Print and shaded views of the part. All mm, measured from the part's lowest x, y and z. Coordinates: 2 decimals unless noted, no trailing zeros. Order: outer loops, then holes, each group sorted by start corner. A loop starts at its lowest first (then second) coordinate and runs counter-clockwise, first axis right, second up.
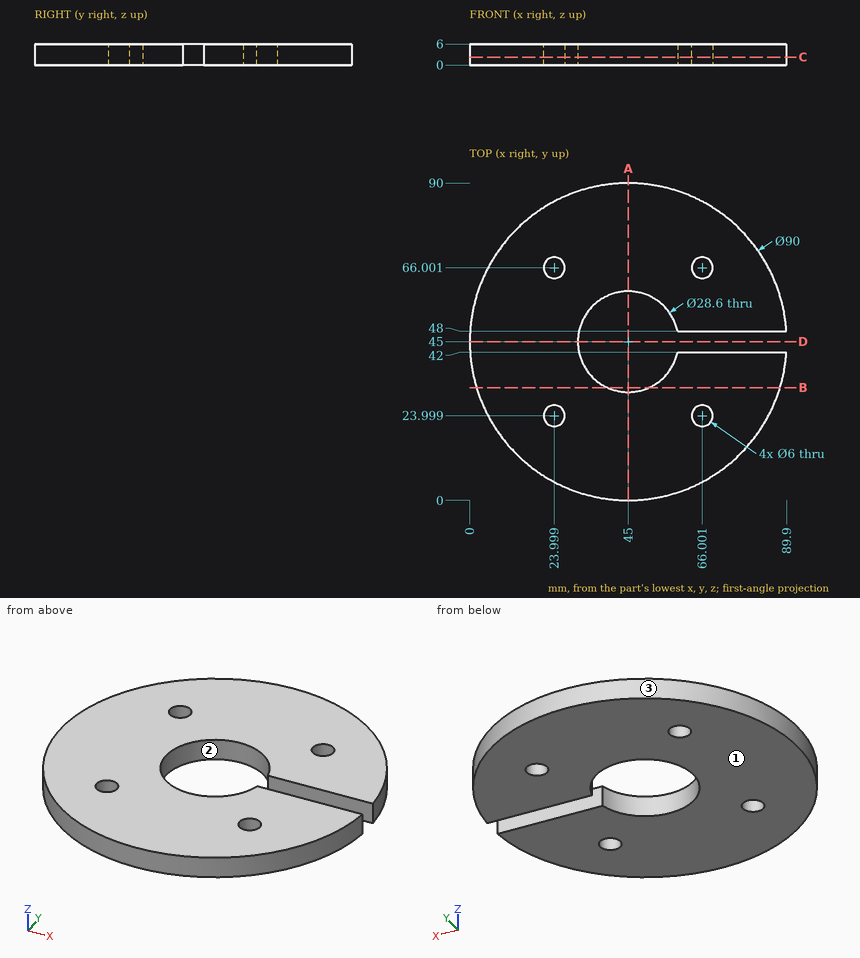
Q1. Mould opens along Y. For the marked faces 1, 2 and 3 say: pulls with the +Y half, pulls with the -Y half, needs draft (parallel to the pull), parting line crosses it, or undercut.
Established:
face 1: needs draft
face 2: undercut
face 3: parting line crosses it
Q2. Cut at A-A, the plane x = 45. List the corners of the cut face in (y, z), plus the area to 3 significant figures.
Established:
outline: (0, 0) - (30.7, 0) - (30.7, 6) - (0, 6) - close; (59.3, 0) - (90, 0) - (90, 6) - (59.3, 6) - close
area: 368 mm2
Q3. Cut at C-C, the plane z = 2.3. List the corners of the cut face in (x, y).
Established:
outline: (58.98, 42) arc R14.3 cw (long way) to (58.98, 48) - (89.9, 48) arc R45 ccw (long way) to (89.9, 42) - close; hole circle Ø6 at (24, 24); hole circle Ø6 at (24, 66); hole circle Ø6 at (66, 24); hole circle Ø6 at (66, 66)
Q4. Cut at D-D, the plane y = 45. List the corners of the cut face in (x, z), plus the area to 3 significant figures.
Established:
outline: (0, 0) - (30.7, 0) - (30.7, 6) - (0, 6) - close
area: 184 mm2
Q5. Cut at B-B, the plane y = 32. List the corners of the cut face in (x, z).
Established:
outline: (1.92, 0) - (39.04, 0) - (39.04, 6) - (1.92, 6) - close; (50.96, 0) - (88.08, 0) - (88.08, 6) - (50.96, 6) - close
Q6. Probe line 1 (X direction, y = 65, z = 0.6); line 2 (X direction, y = 45, z = 3.55); line 3 (Y direction, x = 34.5, z = 3.2). List the from-to ranges inside material, lowest first.
Established:
line 1: x = 4.69 to 21.17, 26.83 to 63.17, 68.83 to 85.31
line 2: x = 0 to 30.7
line 3: y = 1.24 to 35.29, 54.71 to 88.76
Q7. Drop flat-ended pins along their axis: P1, Ø1.8, axis at x = 80.5, z = 3, coming from the -Y side; P2, Ø1.5, axis at x = 78.5, y = 47, coming from the -Z side; P3, Ø3, axis at x = 71, z = 2.5, coming from the +Y side; P4, Ø3, axis at x = 34, z = 4.5, coming from the +Y side. Give the stop position or say it passes through.
Established:
P1: stops at y = 16.23
P2: passes through
P3: stops at y = 82.75
P4: stops at y = 88.99
